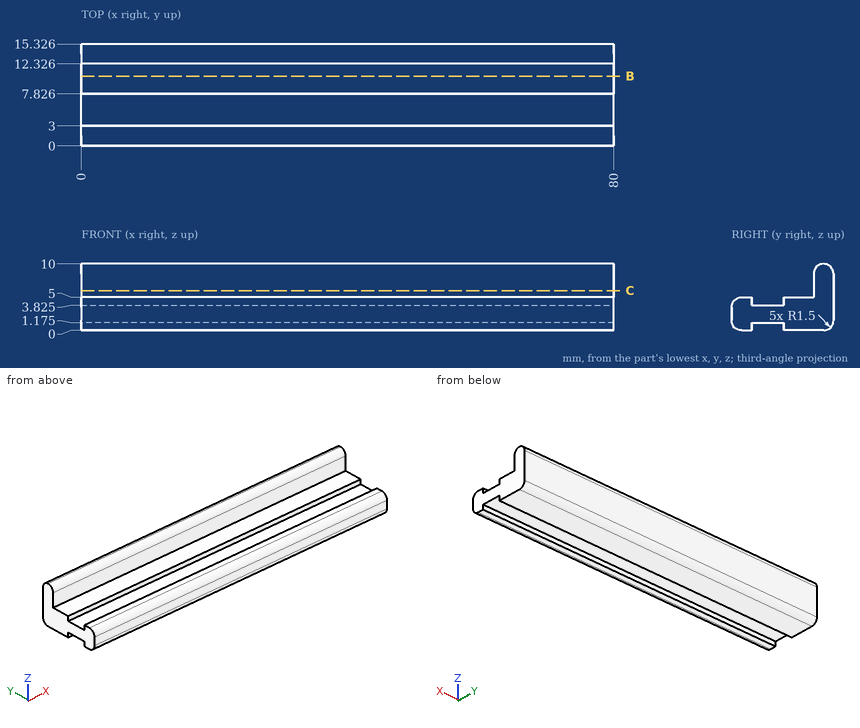
Job drawing, mm, ordinate dimensions from the low corner. One solid piece. Coordinates: 2 decimals unless noted, no trailing zeros. Write each loop counter-clockwise with the first axis right and the second up, starting at its lowest first coordinate (ties: lowest second). Pieces come first, ordered by that corner, then holes.
Item 1: Slice it at C-C (z = 6). Write the cut outline in (x, y).
Item 2: Pin check, flat tips, straight feed: pin 1 (1.2 mm diameter, centred on x = 38.5, y = 2, fed in from +Z); pin 2 (3 mm diameter, centred on x = 15.5, z = 6, fed in from -Y); pin 3 (4 mm diameter, centred on x = 40, y = 5.5, fed in from +Z) (3 decimals). Stop position of each tip, or through.
Item 3: Probe line 1 (Z direction, x = 71, y = 3.5) (3 decimals); line 2 (Y direction, x = 45, z = 0.5); line 3 (Y direction, x = 59.5, z = 8.5). List the from-to ranges inside material, lowest first.
Item 4: Slice it at B-B (y = 10.5). Write the cut outline in (x, z), and give its area (3 significant figures).
Results found:
1. outline: (0, 12.33) - (80, 12.33) - (80, 15.33) - (0, 15.33) - close
2. pin 1: stops at z = 5
2. pin 2: stops at y = 0.38
2. pin 3: stops at z = 3.825
3. line 1: z = 1.175 to 3.825
3. line 2: y = 0.38 to 3, 7.83 to 14.94
3. line 3: y = 12.33 to 15.33
4. outline: (0, 0) - (80, 0) - (80, 5) - (0, 5) - close
4. area: 400 mm2
